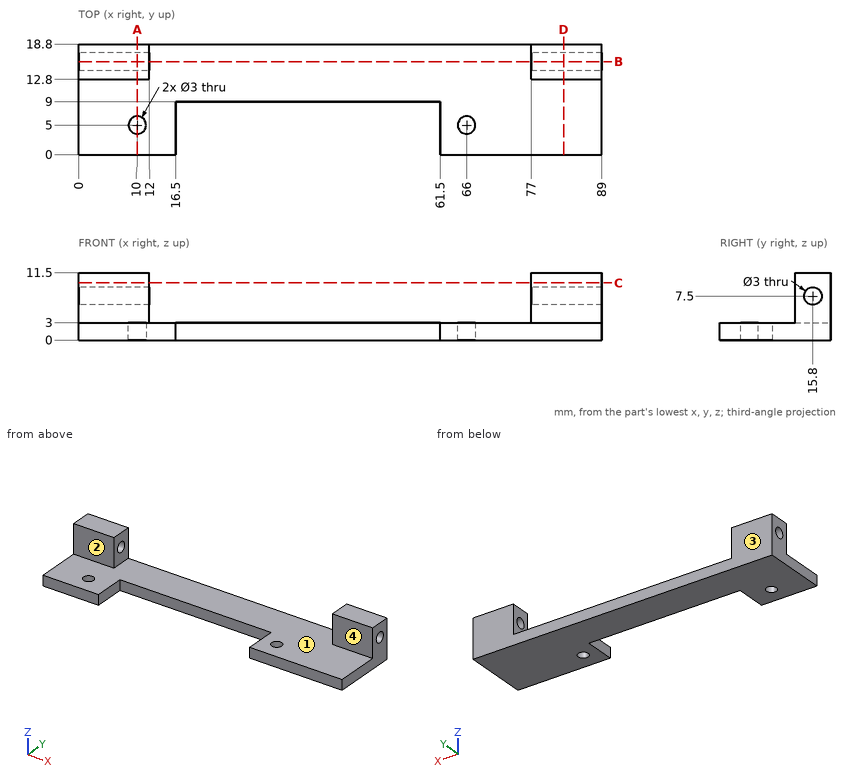
Job drawing, mm, ordinate dimensions from the low corner. One solid piece. A direction names the side the tool comes from. Coordinates: 2 decimals unless noted, no trailing zeros. Order: outer loops, then holes, each group sorted by start corner. A loop starts at its lowest first (then second) coordinate and runs counter-clockwise, first axis right, second up. Notation, with made-up numbers: (-36.5, 52) - (17.5, 52) arc R16 cw to (17.5, 72) - close; hole circle Ø4 at (2.25, 42.5). An arc over 180 degrees is marked (long way). Write each question's results on one line, items separated by ' | '. Start each with the question number.
Item 1: Wall check: probe 1 along X at (y, z) = (16.5, 11); probe 2 along Y at (x, z) = (66, 1.7); probe 3 along Z at (x, y) = (79.5, 15.8). Give the ranges that are in metal, low to high. Write a range as [from, to].
Item 2: Flat gauge pins, fed straight in: pin 1 (5 mm diameter, centred on y = 16, z = 8.5, fed in from +X); pin 2 (5.5 mm diameter, centred on x = 59.5, y = 5, fed in from +Z); pin 3 (2.5 mm diameter, centred on x = 7, z = 8, fed in from -Y); pin 4 (1 mm diameter, centred on x = 32, z = 1.5, fed in from -Y). Where does each tip first touch, or does it go through?
Item 3: Mould opens along X. For the marked faces 1 and 2 say: released by +X, released by -X, zero draft, split by the parting line, or undercut.
Item 4: Band-saw the part on C-C on z = 9.75. Write the cut outline in (x, y), and give its area (3 significant figures).
Item 5: Tool access for the marked faces 3 and 4: list every direction of +Z, -Z, +X, -X, +Y, -Y with a clear straight run to the whole face (end or side of a thin tool).
Item 6: Band-saw the part on A-A on x = 10. Write the cut outline in (y, z), and give its area (3 significant figures).
Item 7: Band-saw the part on B-B on y = 15.8. Write the cut outline in (x, z), and give its area (3 significant figures).
Item 8: Band-saw the part on D-D on x = 82.5. Write the cut outline in (y, z).
Numbers:
1) probe 1: [0, 12], [77, 89] | probe 2: [0, 3.5], [6.5, 18.8] | probe 3: [0, 6], [9, 11.5]
2) pin 1: x = 89 | pin 2: z = 3 | pin 3: y = 12.8 | pin 4: y = 9
3) face 1: undercut | face 2: zero draft
4) outline: (0, 12.8) - (12, 12.8) - (12, 18.8) - (0, 18.8) - close; (77, 12.8) - (89, 12.8) - (89, 18.8) - (77, 18.8) - close | area: 144 mm^2
5) face 3: +Z, -Z, +X, -X, +Y | face 4: +Z, +X, -X, -Y
6) outline: (0, 0) - (3.5, 0) - (3.5, 3) - (0, 3) - close; (6.5, 0) - (18.8, 0) - (18.8, 11.5) - (12.8, 11.5) - (12.8, 3) - (6.5, 3) - close; hole circle Ø3 at (15.8, 7.5) | area: 91.3 mm^2
7) outline: (0, 0) - (89, 0) - (89, 6) - (77, 6) - (77, 3) - (12, 3) - (12, 6) - (0, 6) - close; (0, 9) - (12, 9) - (12, 11.5) - (0, 11.5) - close; (77, 9) - (89, 9) - (89, 11.5) - (77, 11.5) - close | area: 399 mm^2
8) outline: (0, 0) - (18.8, 0) - (18.8, 11.5) - (12.8, 11.5) - (12.8, 3) - (0, 3) - close; hole circle Ø3 at (15.8, 7.5)
